Geometry check sheet. Reference: drawing and pictorial views, mm from the part's lowest x, y, z. A direction names the side the tool comes from. Round coordinates to 2 decimals unless told otherwise and drop trailing zeros. Order: outer loops, then holes, each group sorted by start corner. A loop starts at its lowest first (then second) coordinate and runs counter-clockwise, first axis right, second up.
Q1. Scan lines: probe 1 along Z at (x, y) = (6.35, 5.5) (3 decimals); probe 2 along Z at (x, y) = (6.35, 14.75) (3 decimals); probe 3 along X at (y, z) = (12.5, 6.25). Record each from-to range of solid material in increasing order.
Q2. Cross-section at A-A on x = 6.35. Record the cut outline in (y, z) (3 decimals).
Q3. Cross-section at C-C on z = 4. Record the cut outline in (x, y), then the cut area to 3 significant figures.
Q4. Mould release check, pull along Z, two halves, no side actions. Record for the marked faces 3, 4 and 5: +Z half, -Z half, draft (parallel to the pull), parting line (faces both ways), or undercut.
Q5. Cross-section at B-B on z = 6.35. Give the number of separate pieces and of enclosed holes in the cut face, then the cut area to 3 significant figures.
Q6. Set-up check for the marked faces 1 and 2: record each of +Z, -Z, +X, -X, +Y, -Y from which the full face is reachable in a straight line by a thin tool's end or side.
Q7. Cross-section at D-D on y = 19. Record the cut outline in (x, z) (3 decimals), then the cut area to 3 significant figures.
Q8. Depth check by flat-ended pin: P1, Ø1, axis at x = 8, y = 12.5, coming from the +Z side; P2, Ø3, axis at y = 18.5, z = 9.5, coming from the -X side; P3, Ø1.9, axis at y = 15.24, z = 6.35, coming from the -X side. Enter the tip coordinate at first touch or a pass-through.
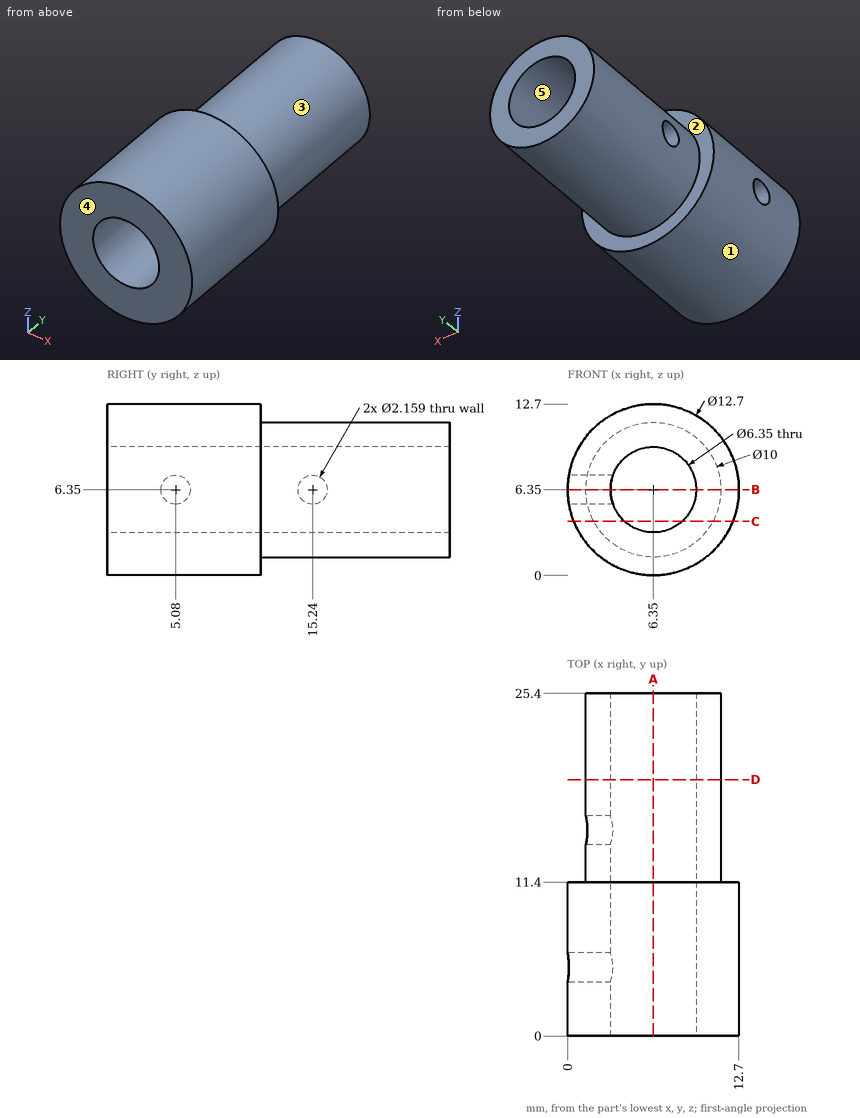
Results found:
1. probe 1: z = 0 to 3.175, 9.525 to 12.7
1. probe 2: z = 1.35 to 3.175, 9.525 to 11.35
1. probe 3: x = 1.35 to 3.18, 9.52 to 11.35
2. outline: (0, 0) - (11.4, 0) - (11.4, 1.35) - (25.4, 1.35) - (25.4, 3.175) - (0, 3.175) - close; (0, 9.525) - (25.4, 9.525) - (25.4, 11.35) - (11.4, 11.35) - (11.4, 12.7) - (0, 12.7) - close
3. outline: (0.45, 0) - (4.22, 0) - (4.22, 25.4) - (1.94, 25.4) - (1.94, 11.4) - (0.45, 11.4) - close; (8.48, 0) - (12.25, 0) - (12.25, 11.4) - (10.76, 11.4) - (10.76, 25.4) - (8.48, 25.4) - close
3. area: 150 mm2
4. face 3: parting line
4. face 4: draft
4. face 5: undercut
5. separate pieces: 4
5. enclosed holes: 0
5. area: 113 mm2
6. face 1: +Y, -Y
6. face 2: +Y
7. outline: circle Ø10 at (6.35, 6.35); hole circle Ø6.35 at (6.35, 6.35)
7. area: 46.9 mm2
8. P1: stops at z = 11.22
8. P2: stops at x = 1.63
8. P3: stops at x = 9.38
